Source: three-view drawing plus pictorial views. Frame: mm from the lowest corner of the part. Give positions to 0.01 mm unless a question says otherwise; leave off trailing zeros. Order: outer loops, then holes, each group sorted by start corner. A loop starts at its lowest first (then second) coordinate and runs counter-clockwise, first axis right, second up. Notation, with made-up numbers: (88, -2.75) -> (92, -2.75) arc R26 cw to (92, 21.25) -> close; hole circle Ø8 at (-32.5, 47.25). An arc over 180 degrees is marked (long way). One line per question, with ' | ' between items.
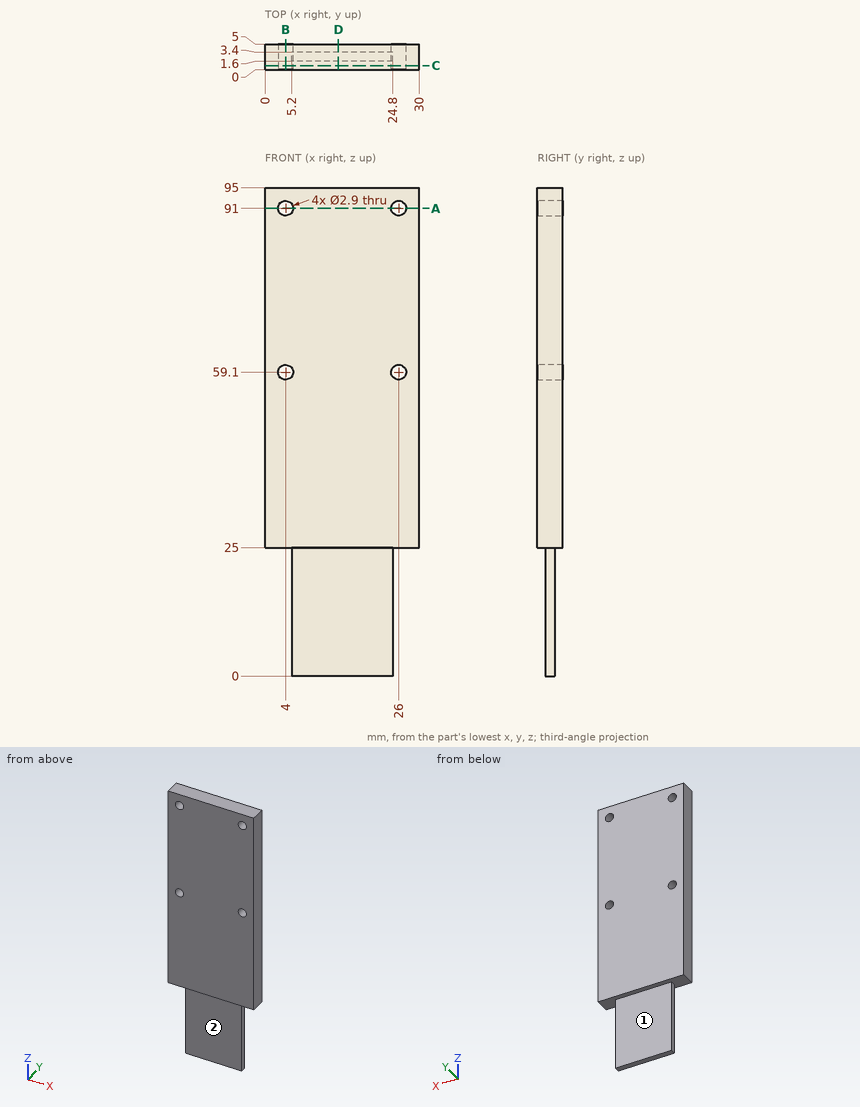
1) Section C-C on y = 0.8. Return loops of the section in (x, z).
Check result:
outline: (0, 25) -> (30, 25) -> (30, 95) -> (0, 95) -> close; hole circle Ø2.9 at (4, 59.1); hole circle Ø2.9 at (4, 91); hole circle Ø2.9 at (26, 59.1); hole circle Ø2.9 at (26, 91)
2) Section D-D on x = 14.25. Return loops of the section in (y, z), plus the area to 3 significant figures.
Check result:
outline: (0, 25) -> (1.6, 25) -> (1.6, 0) -> (3.4, 0) -> (3.4, 25) -> (5, 25) -> (5, 95) -> (0, 95) -> close | area: 395 mm^2
3) Contact query for flat-ended pins moving along their axis: pin 1 Ø2.5 at (x, z) = (26, 91) entering from -Y; pin 2 Ø6 at (x, z) = (11, 14) entering from -Y; pin 3 Ø2 at (y, z) = (2.5, 16) entering from -X; pin 4 Ø1.4 at (y, z) = (2.5, 6.5) entering from +X. Output: stop coordinate, or through.
Check result:
pin 1: passes through | pin 2: stops at y = 1.6 | pin 3: stops at x = 5.2 | pin 4: stops at x = 24.8
4) Section A-A on z = 91. Return loops of the section in (x, y), plus the area to 3 significant figures.
Check result:
outline: (0, 0) -> (2.55, 0) -> (2.55, 5) -> (0, 5) -> close; (5.45, 0) -> (24.55, 0) -> (24.55, 5) -> (5.45, 5) -> close; (27.45, 0) -> (30, 0) -> (30, 5) -> (27.45, 5) -> close | area: 121 mm^2
5) Section B-B on x = 4. Return loops of the section in (y, z), plus the area to 3 significant figures.
Check result:
outline: (0, 25) -> (5, 25) -> (5, 57.65) -> (0, 57.65) -> close; (0, 60.55) -> (5, 60.55) -> (5, 89.55) -> (0, 89.55) -> close; (0, 92.45) -> (5, 92.45) -> (5, 95) -> (0, 95) -> close | area: 321 mm^2
6) Material intervals for probe 1 along Z at (x, y) = (4, 2); probe 2 along X at (y, z) = (1.7, 91); probe 3 along Y at (x, z) = (17, 14), sorted ascending. Write a range as from..to.
Check result:
probe 1: z = 25..57.65, 60.55..89.55, 92.45..95 | probe 2: x = 0..2.55, 5.45..24.55, 27.45..30 | probe 3: y = 1.6..3.4
7) Pull-direction query (Y, two-part tool) for the marked faces 1 and 2; classes: +Y half, -Y half, draft (parallel to the pull), parting line (faces both ways), or undercut.
Check result:
face 1: +Y half | face 2: -Y half
